The listing builds one solid part. Answer for the finished solid, in the listing's coordinates (mm). Face numbers are marked on the shaded views. Give positions to 0.01 mm unless a question says otherwise; leave off trailing zeros. Loops run counter-clockwise (first coordinate to the right, second up) from the corner with the lowest first, then second, coordinate; pieces in that order, holes last. Notation, with made-up numbers: M 10.25,85.25 L 16.25,85.25 A19 cw 16.25,92.25 Z; hole C 69.25,51 d3. An arc over 180 degrees is marked long. Use one line per item in the form item = value. Start each with the question number.
1. Straight lines are drawn through the part: line 1 (Z direction, x = -9.5, y = -0.6); line 2 (X direction, y = -1.35, z = -16.5); line 3 (X direction, y = -1.6, z = -24). For each, find the intervals that lie inside material, in ascending order. Write a range as from..to.
2. The part is cut by section C-C (z = 4). Write down the section's boundary in (x, y), and give its area (3 significant figures).
3. The mould has two halves that part along Z. Classify the marked faces 1 and 2: released by +Z, released by -Z, zero draft, split by the parting line, or undercut.
4. The part is cut by section A-A (x = 0). Write down the section's boundary in (y, z).
5. The part is cut by section B-B (y = 0.7). Write down the section's boundary in (x, z), and give its area (3 significant figures).
6. Each of these flat-tipped pins is pushed along its axis until it touches: pin 1 Ø1.5 at (x, y) = (20, 1) entering from -Z; pin 2 Ø0.8 at (y, z) = (-1, -17.5) entering from +X; pin 3 Ø1 at (y, z) = (1.5, -10) entering from -X. Where does it stop, or does it pass through?
7. The part is cut by section D-D (x = 15). Write down the section's boundary in (y, z).
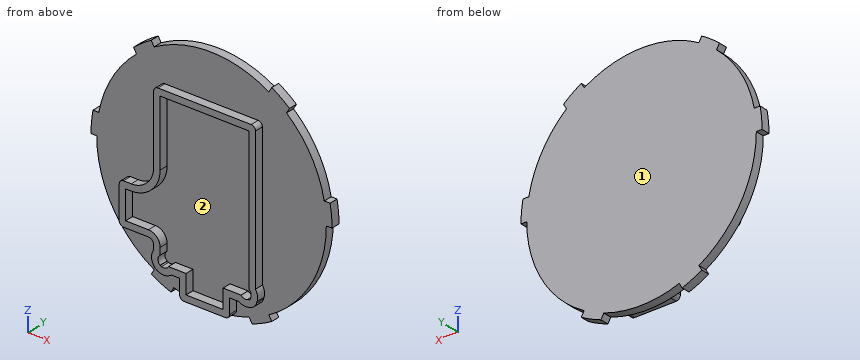
from build123d import *

# Parameters (mm, degrees)
BOSS_EXTRUDE1_DEPTH = 2
BOSS_EXTRUDE2_DEPTH = 2
CUT_EXTRUDE1_DEPTH  = 2
FILLET1_R           = 2
FILLET2_R           = 1


with BuildPart() as part:
    # Sketch1 → Boss-Extrude1 (new body)
    with BuildSketch(Plane(origin=(0, 0, 0), x_dir=(1, 0, 0), z_dir=(0, 1, 0))):
        with BuildLine():
            Line((13.311072252, 23.055453444), (13.974197662, 24.204020346))
            ThreePointArc((13.974197662, 24.204020346), (11.743873388, 25.361274397), (9.418625663, 26.313538185))
            Line((9.418625663, 26.313538185), (8.744070643, 25.145174619))
            ThreePointArc((8.744070643, 25.145174619), (0, 26.622144504), (-8.744070643, 25.145174619))
            Line((-8.744070643, 25.145174619), (-9.418625663, 26.313538185))
            ThreePointArc((-9.418625663, 26.313538185), (-11.743873388, 25.361274397), (-13.974197662, 24.204020346))
            Line((-13.974197662, 24.204020346), (-13.311072252, 23.055453444))
            ThreePointArc((-13.311072252, 23.055453444), (-23.055453444, 13.311072252), (-26.622144504, 0))
            Line((-26.622144504, 0), (-27.948395324, 0))
            ThreePointArc((-27.948395324, 0), (-27.835444594, -2.510144506), (-27.497505363, -5))
            Line((-27.497505363, -5), (-26.148395324, -5))
            ThreePointArc((-26.148395324, -5), (-23.055453444, -13.311072252), (-17.404324681, -20.145174619))
            Line((-17.404324681, -20.145174619), (-18.0788797, -21.313538185))
            ThreePointArc((-18.0788797, -21.313538185), (-16.091571206, -22.851129891), (-13.974197662, -24.204020346))
            Line((-13.974197662, -24.204020346), (-13.311072252, -23.055453444))
            ThreePointArc((-13.311072252, -23.055453444), (0, -26.622144504), (13.311072252, -23.055453444))
            Line((13.311072252, -23.055453444), (13.974197662, -24.204020346))
            ThreePointArc((13.974197662, -24.204020346), (16.091571206, -22.851129891), (18.0788797, -21.313538185))
            Line((18.0788797, -21.313538185), (17.404324681, -20.145174619))
            ThreePointArc((17.404324681, -20.145174619), (23.055453444, -13.311072252), (26.148395324, -5))
            Line((26.148395324, -5), (27.497505363, -5))
            ThreePointArc((27.497505363, -5), (27.835444594, -2.510144506), (27.948395324, 0))
            Line((27.948395324, 0), (26.622144504, 0))
            ThreePointArc((26.622144504, 0), (23.055453444, 13.311072252), (13.311072252, 23.055453444))
        make_face()
    extrude(amount=BOSS_EXTRUDE1_DEPTH)

    # Sketch2 → Boss-Extrude2 (add)
    with BuildSketch(Plane.XZ):
        with BuildLine():
            Line((-5.8, -25.737204514), (5.8, -25.737204514))
            Line((5.8, -25.737204514), (5.8, -21.3))
            Line((5.8, -21.3), (7.903128058, -21.3))
            ThreePointArc((7.903128058, -21.3), (9.07834188, -21.768068718), (10.339619988, -21.671149242))
            ThreePointArc((10.339619988, -21.671149242), (11.075305639, -21.469795949), (11.823980776, -21.323980776))
            ThreePointArc((11.823980776, -21.323980776), (11.969795949, -20.575305639), (12.171149242, -19.839619988))
            ThreePointArc((12.171149242, -19.839619988), (12.268068718, -18.57834188), (11.8, -17.403128058))
            Line((11.8, -17.403128058), (11.8, 16.3))
            Line((11.8, 16.3), (-11.8, 16.3))
            Line((-11.8, 16.3), (-11.8, -0.5))
            ThreePointArc((-11.8, -0.5), (-13.323044738, -4.176955262), (-17, -5.7))
            Line((-17, -5.7), (-19.8, -5.7))
            Line((-19.8, -5.7), (-19.8, -15.3))
            Line((-19.8, -15.3), (-13, -15.3))
            ThreePointArc((-13, -15.3), (-12.151471863, -15.651471863), (-11.8, -16.5))
            Line((-11.8, -16.5), (-11.8, -17.563099043))
            ThreePointArc((-11.8, -17.563099043), (-12.3, -19.159970985), (-11.8, -20.756842927))
            Line((-11.8, -20.756842927), (-11.8, -21.343991953))
            ThreePointArc((-11.8, -21.343991953), (-11.166576007, -21.530222711), (-10.546527145, -21.757042593))
            ThreePointArc((-10.546527145, -21.757042593), (-9.056966413, -21.924699044), (-7.694376613, -21.3))
            Line((-7.694376613, -21.3), (-5.8, -21.3))
            Line((-5.8, -21.3), (-5.8, -25.737204514))
        make_face()
    extrude(amount=BOSS_EXTRUDE2_DEPTH)

    # Sketch4 → Cut-Extrude1 (cut)
    with BuildSketch(Plane.XZ.offset(2)):
        with BuildLine():
            Line((-4.3, -19.8), (-4.3, -24.237204514))
            Line((-4.3, -24.237204514), (4.3, -24.237204514))
            Line((4.3, -24.237204514), (4.3, -19.8))
            Line((4.3, -19.8), (8.475304923, -19.8))
            ThreePointArc((8.475304923, -19.8), (9.113730299, -20.241287927), (9.889823566, -20.240176434))
            ThreePointArc((9.889823566, -20.240176434), (10.220030244, -20.141701714), (10.552993589, -20.052993589))
            ThreePointArc((10.552993589, -20.052993589), (10.641701714, -19.720030244), (10.740176434, -19.389823566))
            ThreePointArc((10.740176434, -19.389823566), (10.741287927, -18.613730299), (10.3, -17.975304923))
            Line((10.3, -17.975304923), (10.3, 14.8))
            Line((10.3, 14.8), (-10.3, 14.8))
            Line((-10.3, 14.8), (-10.3, -0.5))
            ThreePointArc((-10.3, -0.5), (-12.262384566, -5.237615434), (-17, -7.2))
            Line((-17, -7.2), (-18.3, -7.2))
            Line((-18.3, -7.2), (-18.3, -13.8))
            Line((-18.3, -13.8), (-13, -13.8))
            ThreePointArc((-13, -13.8), (-11.090811691, -14.590811691), (-10.3, -16.5))
            Line((-10.3, -16.5), (-10.3, -18.135275908))
            ThreePointArc((-10.3, -18.135275908), (-10.8, -19.159970985), (-10.3, -20.184666062))
            Line((-10.3, -20.184666062), (-10.3, -20.244402637))
            ThreePointArc((-10.3, -20.244402637), (-10.1425072, -20.303948315), (-9.985887603, -20.365754231))
            ThreePointArc((-9.985887603, -20.365754231), (-9.070775843, -20.387067812), (-8.368468799, -19.8))
            Line((-8.368468799, -19.8), (-4.3, -19.8))
        make_face()
    extrude(amount=-CUT_EXTRUDE1_DEPTH, mode=Mode.SUBTRACT)

    # Fillet1
    # the kernel refuses this fillet: 2 mm, written as the material it takes off along each edge
    with BuildSketch(Plane(origin=(11.823980776, 0, -21.323980776), x_dir=(0.21089533444820466, 0, 0.977508648508022), z_dir=(0, -1, 0))) as fillet1_piece_1:
        with BuildLine():
            CenterArc((1.288021457, 1.996690902), FILLET1_R, 207.646032977, 59.057586609)
            Line((-0.48364068, 1.068675131), (-0.519073923, 1.050114816))
            ThreePointArc((-0.519073923, 1.050114816), (-0.262887012, 0.524803612), (-0.037329873, -0.014369433))
            Line((-0.037329873, -0.014369433), (0.002300038, -0.039933818))
            ThreePointArc((0.002300038, -0.039933818), (0.586509771, -0.023123602), (1.170719503, -0.039933818))
            Line((1.170719503, -0.039933818), (1.173019541, 0))
        make_face()
    extrude(amount=4.932548853, mode=Mode.SUBTRACT)
    with BuildSketch(Plane(origin=(-11.8, 0, -21.343991953), x_dir=(0.9530196078830334, 0, -0.3029086116149048), z_dir=(0, -1, 0))) as fillet1_piece_2:
        with BuildLine():
            CenterArc((1.212682202, 1.99706697), FILLET1_R, 225.951474685, 40.945152222)
            Line((-0.177852496, 0.559564534), (-0.20566319, 0.530814485))
            ThreePointArc((-0.20566319, 0.530814485), (-0.127047032, 0.267665923), (-0.038120784, -0.012116344))
            Line((-0.038120784, -0.012116344), (0.002165504, -0.039941339))
            ThreePointArc((0.002165504, -0.039941339), (0.552203503, -0.025041546), (1.102241502, -0.039941339))
            Line((1.102241502, -0.039941339), (1.104407006, 0))
        make_face()
    extrude(amount=4.761017514, mode=Mode.SUBTRACT)

    # Fillet2
    fillet2_edges = [part.edges().sort_by_distance(p)[0] for p in [
        (-5.8, -1, -25.737204514),
        (5.8, -1, -25.737204514),
        (11.8, -1, 16.3),
        (-11.8, -1, 16.3),
        (-19.8, -1, -5.7),
        (-19.8, -1, -15.3),
    ]]
    fillet(fillet2_edges, radius=FILLET2_R)


solid = part.part
Derived:
q1.line_1 = -21.96..-20.46, 14.8..16.3
q1.line_2 = -11.8..-10.3, 10.3..11.8
q1.line_3 = -5.8..-4.3, 4.3..5.8
q2.outline = M -27.66,0 L -11.8,0 L -11.8,-2 L -10.3,-2 L -10.3,0 L 10.3,0 L 10.3,-2 L 11.8,-2 L 11.8,0 L 27.66,0 L 27.66,2 L -27.66,2 Z
q2.area = 117 mm2
q3.face_1 = zero draft
q3.face_2 = undercut
q4.outline = M -2,-25.74 L 0,-25.74 L 0,-26.62 L 2,-26.62 L 2,26.62 L 0,26.62 L 0,16.3 L -2,16.3 L -2,14.8 L 0,14.8 L 0,-24.24 L -2,-24.24 Z
q5.outline = M -27.95,0 L -26.62,0 A26.62 ccw -13.31,-23.06 L -13.97,-24.2 A27.95 ccw -9.42,-26.31 L -8.74,-25.15 A26.62 ccw 8.74,-25.15 L 9.42,-26.31 A27.95 ccw 13.97,-24.2 L 13.31,-23.06 A26.62 ccw 26.62,0 L 27.95,0 A27.95 ccw 27.5,5 L 26.15,5 A26.62 ccw 17.4,20.15 L 18.08,21.31 A27.95 ccw 13.97,24.2 L 13.31,23.06 A26.62 ccw -13.31,23.06 L -13.97,24.2 A27.95 ccw -18.08,21.31 L -17.4,20.15 A26.62 ccw -26.15,5 L -27.5,5 A27.95 ccw Z
q5.area = 2,270 mm2
q6.pin_1 = -18.39
q6.pin_2 = 12.07
q6.pin_3 = -24.87
q7.outline = M 0,-21.99 L 2,-21.99 L 2,23.58 L 0,23.58 Z
